from build123d import *

# Parameters (mm, degrees)
F0_R     = 2.54
F1_DEPTH = 8.89
F2_R     = 5.08
F2_R_2   = 2.54
F3_DEPTH = 2.54
F4_R     = 1.262095
F5_DEPTH = 25.4


with BuildPart() as f1:
    # F0 (on Top) → F1 (new body)
    with BuildSketch(Plane.XY):
        Circle(F0_R)
    extrude(amount=F1_DEPTH)

    # F2 (on face) → F3 (join)
    with BuildSketch(Plane(origin=(0, 0, 0), x_dir=(1, 0, 0), z_dir=(0, 0, -1))):
        Circle(F2_R)
        Circle(F2_R_2, mode=Mode.SUBTRACT)
    extrude(amount=-F3_DEPTH)

    # F4 (on face) → F5 (cut)
    with BuildSketch(Plane(origin=(0, 0, 0), x_dir=(1, 0, 0), z_dir=(0, 0, -1))):
        Circle(F4_R)
    extrude(amount=-F5_DEPTH, mode=Mode.SUBTRACT)


solid = f1.part
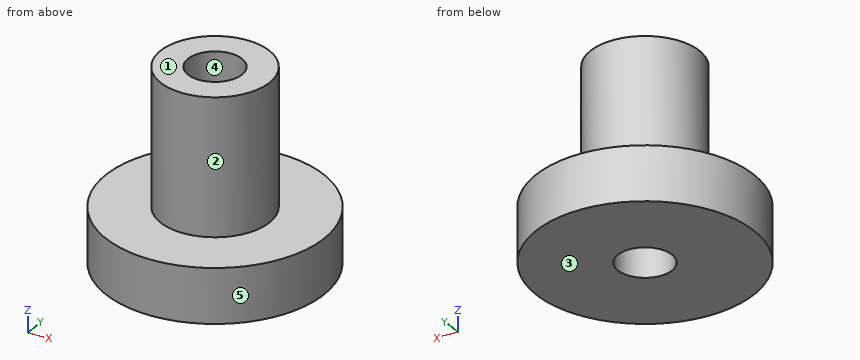
Could you check a few things on this model? Use its own coordinates, in mm. Face numbers are marked on the shaded views. A direction names the side the tool comes from. Coordinates: 2 decimals unless noted, no trailing zeros. Order: outer loops, then holes, each group sorted by start corner. A loop starts at its lowest first (then second) coordinate and runs counter-clockwise, first axis right, second up. Notation, with made-up numbers: (-36.75, 74.5) - (0.25, 74.5) arc R7 ccw to (0.25, 86.5) - close; hole circle Ø7 at (26, 55). An arc over 180 degrees is marked (long way). Answer in a Markdown table with one row per item. Add a question column.
(1) If we section it at C-C, the plane z = 3.75: Please give me the cut outline in (x, y), then the cut area to 3 significant figures.
(2) If we section it at A-A, the plane x = 0: Please give me the cut outline in (y, z).
(3) If we section it at D-D, the plane y = -1.5: Please give me the cut outline in (x, z), then the cut area to 3 significant figures.
(4) On a 3-axis mill with a long thin cutter (end or side, diameter ignored), from which of +Z, -Z, +X, -X, +Y, -Y can I reach the whole of each face in a straight line? I mean the marked faces 1 and 2. Say none if no direction works.
(5) If we mould it in two halves opening along X, with no side actions, what happens to the marked faces 3, 4 and 5? For each: released by +X, released by -X, zero draft, split by the parting line, or undercut.
(6) I need wall thicknesses on L1, parallel to Y at x = 0, z = 2.25; L2, parallel to X at y = 0, z = 6.5. Which ranges of each line are inside material? Lowest first, please.
(7) Will these pins go through, and if not, where does the flat tip stop? pin 1 (4 mm diameter, centred on y = -2, z = 5.5, fed in from +X); pin 2 (1 mm diameter, centred on x = -0.5, y = -3.5, fed in from +Z); pin 3 (3 mm diameter, centred on x = 3.5, z = 3, fed in from -Y).
Results are:
| question | item | result |
|---|---|---|
| 1 | outline | circle Ø5.08 at (0, 0); hole circle Ø2.52 at (0, 0) |
| 1 | area | 15.3 mm2 |
| 2 | outline | (-5.08, 0) - (-1.26, 0) - (-1.26, 8.89) - (-2.54, 8.89) - (-2.54, 2.54) - (-5.08, 2.54) - close; (1.26, 0) - (5.08, 0) - (5.08, 2.54) - (2.54, 2.54) - (2.54, 8.89) - (1.26, 8.89) - close |
| 3 | outline | (-4.85, 0) - (4.85, 0) - (4.85, 2.54) - (2.05, 2.54) - (2.05, 8.89) - (-2.05, 8.89) - (-2.05, 2.54) - (-4.85, 2.54) - close |
| 3 | area | 50.7 mm2 |
| 4 | face 1 | +Z, +X, -X, +Y, -Y |
| 4 | face 2 | +Z |
| 5 | face 3 | zero draft |
| 5 | face 4 | undercut |
| 5 | face 5 | split by the parting line |
| 6 | L1 | y = -5.08 to -1.26, 1.26 to 5.08 |
| 6 | L2 | x = -2.54 to -1.26, 1.26 to 2.54 |
| 7 | pin 1 | stops at x = 2.54 |
| 7 | pin 2 | stops at z = 2.54 |
| 7 | pin 3 | stops at y = -4.64 |
